```python
from build123d import *

# Parameters (mm, degrees)
F0_W      = 28.575
F0_H      = 25.4
F1_DEPTH  = 25.4
F2_R      = 5.08
F3_W      = 12.7
F3_H      = 4.7625
F4_DEPTH  = 12.7
F5_W      = 11.1125
F5_H      = 1.5875
F6_DEPTH  = 10.922
F7_W      = 1.5875
F7_H      = 6.35
F8_DEPTH  = 9.525
F9_W      = 6.35
F9_H      = 3.1623
F10_DEPTH = 1.5875
F11_R     = 1.5875
F12_DEPTH = 1.5875
F13_R     = 5.08
F14_W     = 1.5875
F14_H     = 6.35
F15_DEPTH = 9.525
F16_W     = 6.35
F16_H     = 3.175
F17_DEPTH = 1.5875
F18_R     = 1.5875
F19_DEPTH = 1.5875
F20_R     = 5.08
F21_SIZE  = 0.254
F22_SIZE  = 0.254


with BuildPart() as f1:
    # F0 (on Top) → F1 (new body)
    with BuildSketch(Plane.XY):
        with Locations((14.2875, -12.7)):
            Rectangle(F0_W, F0_H)
    extrude(amount=F1_DEPTH)

    # F2
    f2_edges = [f1.edges().sort_by_distance(p)[0] for p in [
        (14.2875, -25.4, 25.4),
        (14.2875, 0, 25.4),
        (14.2875, -25.4, 0),
        (14.2875, 0, 0),
    ]]
    fillet(f2_edges, radius=F2_R)

    # F3 (on face) → F4 (cut)
    with BuildSketch(Plane.YZ.offset(28.575)):
        with Locations((-12.7, 16.66875)):
            Rectangle(F3_W, F3_H)
    extrude(amount=-F4_DEPTH, mode=Mode.SUBTRACT)

    # F5 (on face) → F6 (join)
    with BuildSketch(Plane.YZ.offset(15.875)):
        with Locations((-12.69365, 15.8069642857)):
            Rectangle(F5_W, F5_H)
    extrude(amount=F6_DEPTH)

    # F7 (on face) → F8 (join)
    with BuildSketch(Plane(origin=(0, 0, 0), x_dir=(0, -1, 0), z_dir=(-1, 0, 0))):
        with Locations((19.84375, 12.7)):
            Rectangle(F7_W, F7_H)
    extrude(amount=F8_DEPTH)

    # F9 (on face) → F10 (join)
    with BuildSketch(Plane.XZ.offset(20.6375)):
        Polygon((-15.875, 11.1125), (-9.525, 9.525), (-9.525, 11.1125), align=None)
        with Locations((-12.7, 12.69365)):
            Rectangle(F9_W, F9_H)
        Polygon((-15.875, 14.2748), (-9.525, 14.2748), (-9.525, 15.875), align=None)
    extrude(amount=-F10_DEPTH)

    # F11 (on face) → F12 (cut)
    with BuildSketch(Plane.XZ.offset(20.6375)):
        with Locations((-11.1124364053, 12.7375950676)):
            Circle(F11_R)
    extrude(amount=-F12_DEPTH, mode=Mode.SUBTRACT)

    # F13
    f13_edges = [f1.edges().sort_by_distance(p)[0] for p in [
        (-9.525, -19.84375, 15.875),
        (-9.525, -19.84375, 9.525),
    ]]
    fillet(f13_edges, radius=F13_R)

    # F14 (on face) → F15 (join)
    with BuildSketch(Plane(origin=(0, 0, 0), x_dir=(0, -1, 0), z_dir=(-1, 0, 0))):
        with Locations((7.14375, 12.7)):
            Rectangle(F14_W, F14_H)
    extrude(amount=F15_DEPTH)

    # F16 (on face) → F17 (join)
    with BuildSketch(Plane.XZ.offset(7.9375)):
        with Locations((-12.7, 12.7)):
            Rectangle(F16_W, F16_H)
        Polygon((-9.525, 14.2875), (-9.525, 15.875), (-15.875, 14.2875), align=None)
        Polygon((-9.525, 9.525), (-9.525, 11.1125), (-15.875, 11.1125), align=None)
    extrude(amount=-F17_DEPTH)

    # F18 (on face) → F19 (cut)
    with BuildSketch(Plane.XZ.offset(7.9375)):
        with Locations((-11.1125, 12.7)):
            Circle(F18_R)
    extrude(amount=-F19_DEPTH, mode=Mode.SUBTRACT)

    # F20
    f20_edges = [f1.edges().sort_by_distance(p)[0] for p in [
        (-9.525, -7.14375, 15.875),
        (-9.525, -7.14375, 9.525),
    ]]
    fillet(f20_edges, radius=F20_R)

    # F21
    f21_edges = [f1.edges().sort_by_distance(p)[0] for p in [
        (28.575, -12.7, 25.4),
    ]]
    chamfer(f21_edges, length=F21_SIZE)

    # F22
    f22_edges = [f1.edges().sort_by_distance(p)[0] for p in [
        (0, -12.7, 25.4),
    ]]
    chamfer(f22_edges, length=F22_SIZE)


solid = f1.part
```
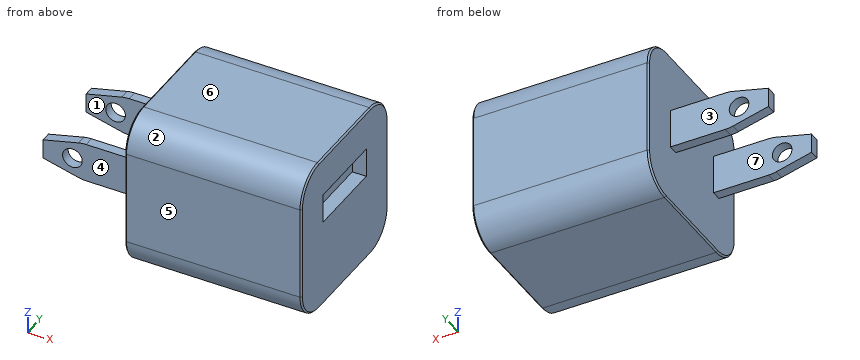
The listing builds one solid part. Answer for the finished solid, in the listing's coordinates (mm). Face numbers are marked on the shaded views. A direction names the side the tool comes from. Give positions to 0.01 mm unless a question says otherwise; leave off trailing zeros. Write each loop counter-clockwise with the first axis right and the second up, starting at its lowest first coordinate (ties: lowest second). Pieces come first, ordered by that corner, then holes. Notation, with made-up numbers: (-7, 87.25) -> (46, 87.25) arc R6 cw to (46, 92.25) -> close; hole circle Ø2 at (-37, 43). An arc over 180 degrees is marked (long way). Write item = value, one per line. Start each with the question number.
1) The part is cut by section C-C, the plane z = 18.5. Determine the outline of the cut face in (x, y) (3 decimals).
2) Determine the mould class of the marked faces 5, 6 and 7 for opening direction Y: +Y half, -Y half, draft (parallel to the pull), parting line (faces both ways), or undercut.
3) Each of these flat-tipped pins is pushed along its axis until it touches: pin 1 (2 mm diameter, centred on y = -20.5, z = 5.5, fed in from -X); pin 2 (4 mm diameter, centred on x = -11.11, z = 12.74, fed in from -Y); pin 3 (7 mm diameter, centred on x = -10.5, z = 13, fed in from +Y). Where does it stop, or does it pass through?
4) Straight lines are drawn through the part: line 1 along Z through (x, y) = (25, -17); line 2 along Y through (x, z) = (-2.5, 12.5); line 3 along X through (y, z) = (-23.5, 15.75) (3 decimals). For each, find the intervals that lie inside material, in ascending order.
5) The part is cut by section A-A, the plane x = 23.5. Determine the outline of the cut face in (y, z).
6) Which of the six approach directions +Z, -Z, +X, -X, +Y, -Y give full straight-line access (tool end or side, diameter ignored) to the marked faces 1, 2, 3 and 4?
7) The part is cut by section D-D, the plane x = 8.5. Determine the outline of the cut face in (y, z).
Solutions:
q1.outline = (0, -25.146) -> (0.254, -25.4) -> (28.321, -25.4) -> (28.575, -25.146) -> (28.575, -19.05) -> (15.875, -19.05) -> (15.875, -6.35) -> (28.575, -6.35) -> (28.575, -0.254) -> (28.321, 0) -> (0.254, 0) -> (0, -0.254) -> close
q2.face_5 = -Y half
q2.face_6 = draft
q2.face_7 = undercut
q3.pin_1 = 0
q3.pin_2 = -20.64
q3.pin_3 = -6.35
q4.line_1 = 0 to 14.29, 15.01 to 16.6, 19.05 to 25.4
q4.line_2 = -20.64 to -19.05, -7.94 to -6.35
q4.line_3 = 0 to 28.575
q5.outline = (-25.4, 5.08) arc R5.08 ccw to (-20.32, 0) -> (-5.08, 0) arc R5.08 ccw to (0, 5.08) -> (0, 20.32) arc R5.08 ccw to (-5.08, 25.4) -> (-20.32, 25.4) arc R5.08 ccw to (-25.4, 20.32) -> close; (-18.25, 15.01) -> (-7.14, 15.01) -> (-7.14, 16.6) -> (-18.25, 16.6) -> close; hole (-19.05, 14.29) -> (-6.35, 14.29) -> (-6.35, 19.05) -> (-19.05, 19.05) -> close
q6.face_1 = +Z, -Z, -X
q6.face_2 = +Z, +X, -X, -Y
q6.face_3 = +Z, -Z, -X, +Y
q6.face_4 = +Z, -Z, -X, -Y
q7.outline = (-25.4, 5.08) arc R5.08 ccw to (-20.32, 0) -> (-5.08, 0) arc R5.08 ccw to (0, 5.08) -> (0, 20.32) arc R5.08 ccw to (-5.08, 25.4) -> (-20.32, 25.4) arc R5.08 ccw to (-25.4, 20.32) -> close
